For this review, take the finished solid that the model builds, in its own axes (mm). Coordinates: 2 decimals unless noted, no trailing zeros. Loops run counter-clockwise (first coordinate to the right, second up) from the corner with the lowest first, then second, coordinate; pieces in that order, holes last. Notation, with made-up numbers: (-35.75, 7.25) -> (2.25, 7.25) arc R32 ccw to (2.25, 43.25) -> close; hole circle Ø3 at (-29.5, 68). An arc over 180 degrees is marked (long way). Use a Markdown table: item, result.
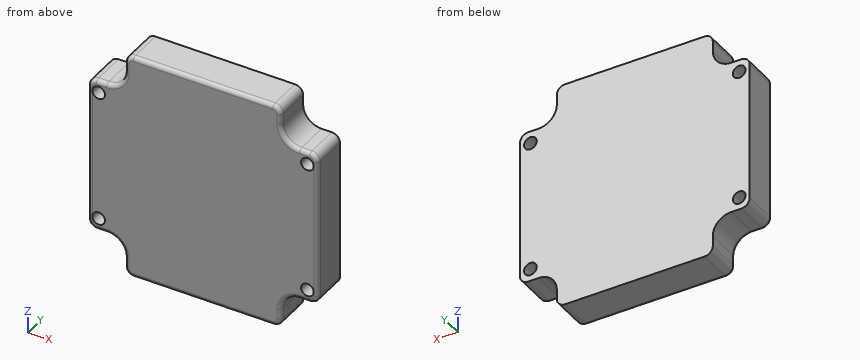
from build123d import *

# Parameters (mm, degrees)
F0_R     = 1.55
F1_DEPTH = 9
F2_R     = 0.99999


# Not quite as in the source:
# - a fillet or chamfer is up to 0.001 mm smaller than in the source, because OpenCascade refuses the exact size


with BuildPart() as f1:
    # F0 (on Front) → F1 (new body)
    with BuildSketch(Plane.XZ):
        with BuildLine():
            Line((17.05, 28), (-17.05, 28))
            ThreePointArc((-17.05, 28), (-18.4642135624, 27.4142135624), (-19.05, 26))
            Line((-19.05, 26), (-19.05, 23.5))
            ThreePointArc((-19.05, 23.5), (-20.3680194847, 20.3180194847), (-23.55, 19))
            Line((-23.55, 19), (-26.05, 19))
            ThreePointArc((-26.05, 19), (-27.4642135624, 18.4142135624), (-28.05, 17))
            Line((-28.05, 17), (-28.05, -17))
            ThreePointArc((-28.05, -17), (-27.4642135624, -18.4142135624), (-26.05, -19))
            Line((-26.05, -19), (-23.55, -19))
            ThreePointArc((-23.55, -19), (-20.3680194847, -20.3180194847), (-19.05, -23.5))
            Line((-19.05, -23.5), (-19.05, -26))
            ThreePointArc((-19.05, -26), (-18.4642135624, -27.4142135624), (-17.05, -28))
            Line((-17.05, -28), (17.05, -28))
            ThreePointArc((17.05, -28), (18.4642135624, -27.4142135624), (19.05, -26))
            Line((19.05, -26), (19.05, -23.5))
            ThreePointArc((19.05, -23.5), (20.3680194847, -20.3180194847), (23.55, -19))
            Line((23.55, -19), (26.05, -19))
            ThreePointArc((26.05, -19), (27.4642135624, -18.4142135624), (28.05, -17))
            Line((28.05, -17), (28.05, 17))
            ThreePointArc((28.05, 17), (27.4642135624, 18.4142135624), (26.05, 19))
            Line((26.05, 19), (23.55, 19))
            ThreePointArc((23.55, 19), (20.3680194847, 20.3180194847), (19.05, 23.5))
            Line((19.05, 23.5), (19.05, 26))
            ThreePointArc((19.05, 26), (18.4642135624, 27.4142135624), (17.05, 28))
        make_face()
        with Locations((-25.5, -16)):
            Circle(F0_R, mode=Mode.SUBTRACT)
        with Locations((25.5, -16)):
            Circle(F0_R, mode=Mode.SUBTRACT)
        with Locations((-25.5, 16)):
            Circle(F0_R, mode=Mode.SUBTRACT)
        with Locations((25.5, 16)):
            Circle(F0_R, mode=Mode.SUBTRACT)
    extrude(amount=F1_DEPTH)

    # F2 (radius 1 in the source; OpenCascade refuses exactly that, so slightly less here)
    f2_edges = [f1.edges().sort_by_distance(p)[0] for p in [
        (-27.464214, -9, 18.414214),
    ]]
    fillet(f2_edges, radius=F2_R)


solid = f1.part
(1) Take a section at A-A on z = 16. State how many separate pieces and enclosed holes the cut face has, plus the area to 3 significant figures.
Found:
| item | result |
|---|---|
| separate pieces | 3 |
| enclosed holes | 0 |
| area | 449 mm^2 |
(2) Take a section at B-B on y = -5.25. Write out the cut boundary in (x, z), plus the area to 3 significant figures.
Found:
| item | result |
|---|---|
| outline | (-28.05, -17) arc R2 ccw to (-26.05, -19) -> (-23.55, -19) arc R4.5 cw to (-19.05, -23.5) -> (-19.05, -26) arc R2 ccw to (-17.05, -28) -> (17.05, -28) arc R2 ccw to (19.05, -26) -> (19.05, -23.5) arc R4.5 cw to (23.55, -19) -> (26.05, -19) arc R2 ccw to (28.05, -17) -> (28.05, 17) arc R2 ccw to (26.05, 19) -> (23.55, 19) arc R4.5 cw to (19.05, 23.5) -> (19.05, 26) arc R2 ccw to (17.05, 28) -> (-17.05, 28) arc R2 ccw to (-19.05, 26) -> (-19.05, 23.5) arc R4.5 cw to (-23.55, 19) -> (-26.05, 19) arc R2 ccw to (-28.05, 17) -> close; hole circle Ø3.1 at (-25.5, -16); hole circle Ø3.1 at (-25.5, 16); hole circle Ø3.1 at (25.5, -16); hole circle Ø3.1 at (25.5, 16) |
| area | 2,800 mm^2 |
(3) For pin 1 Ø1.2 at (y, z) = (-4, 24.5) entering from +X; pin 2 Ø1.9 at (x, z) = (25.5, 16) entering from +Y; pin 3 Ø2 at (x, y) = (-25, -4) entering from +Z; pin 4 Ø3 at (x, y) = (-25, -5) entering from -Z, all flat-tipped, find the tip position at first contact; note any pin that passes through.
Found:
| item | result |
|---|---|
| pin 1 | stops at x = 19.05 |
| pin 2 | passes through |
| pin 3 | stops at z = 19 |
| pin 4 | stops at z = -19 |
(4) For line 1 along Z through (x, y) = (25.5, -5.75); line 2 along X through (y, z) = (-8.5, -15.5); line 3 along X through (y, z) = (-8.5, -21), list the stretches that pass through material, from the lowest coordinate up.
Found:
| item | result |
|---|---|
| line 1 | z = -19 to -17.55, -14.45 to 14.45, 17.55 to 19 |
| line 2 | x = -27.92 to -26.97, -24.03 to 24.03, 26.97 to 27.92 |
| line 3 | x = -19.65 to 19.65 |
